from build123d import *

# Parameters (mm, degrees)
SKETCH1_R           = 3
BOSS_EXTRUDE1_DEPTH = 27
SKETCH2_R           = 4
BOSS_EXTRUDE2_DEPTH = 4
CHAMFER1_SIZE       = 2


with BuildPart() as part:
    # Sketch1 → Boss-Extrude1 (new body)
    with BuildSketch(Plane(origin=(0, 0, 0), x_dir=(0, 0, -1), z_dir=(1, 0, 0))):
        Circle(SKETCH1_R)
    extrude(amount=BOSS_EXTRUDE1_DEPTH)

    # Sketch2 → Boss-Extrude2 (add)
    with BuildSketch(Plane.ZY):
        Circle(SKETCH2_R)
    extrude(amount=BOSS_EXTRUDE2_DEPTH)

    # Chamfer1
    chamfer1_edges = [part.edges().sort_by_distance(p)[0] for p in [
        (-4, 0, -4),
    ]]
    chamfer(chamfer1_edges, length=CHAMFER1_SIZE)


solid = part.part
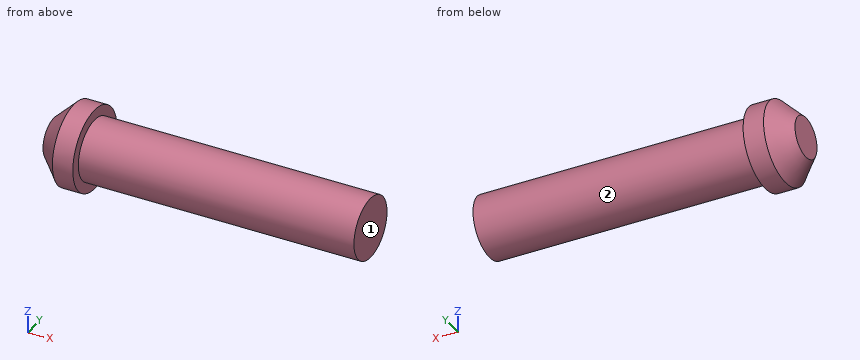
Geometry check sheet. Reference: the model listing, model coordinates, mm. Face numbers are marked on the shaded views. A direction names the side the tool comes from. Round coordinates to 2 decimals unless told otherwise and drop trailing zeros. Loops run counter-clockwise (first coordinate to the right, second up) from the corner with the lowest first, then second, coordinate; pieces in that order, holes last. Notation, with made-up numbers: (84, 22.25) - (116, 22.25) arc R7 ccw to (116, 28.25) - close; hole circle Ø8 at (-38, 32.5). An arc over 180 degrees is marked (long way). One line per question, with ' | ' between items. Start each with the question number.
1. Scan lines: line 1 (Z direction, x = -1.5, y = 3.5); line 2 (Y direction, x = -2.5, z = -1.25); line 3 (X direction, y = -2.75, z = 2.25). Record each from-to range of solid material in increasing order. Write a range as [from, to].
2. Depth check by flat-ended pin: pin 1 (1.5 mm diameter, centred on x = 19, z = 0, fed in from -Y); pin 2 (1.5 mm diameter, centred on x = 2.5, y = -3, fed in from -Z); pin 3 (4 mm diameter, centred on x = 23.5, y = 2.5, fed in from +Z). Enter the tip coordinate at first touch or a pass-through.
3. Tool access check on the marked faces 1 and 2. Record the directions out of +Z, -Z, +X, -X, +Y, -Y that give a thin tool (end or side, any length) a straight path to the whole face; none if there is none.
4. Cross-section at A-A on z = 0. Record the cut outline in (x, y), then the cut area to 3 significant figures.
5. Cross-section at C-C on x = 6. Record the cut outline in (y, z).
Taken from the geometry:
1) line 1: [-1.94, 1.94] | line 2: [-3.27, 3.27] | line 3: [-2.45, 0]
2) pin 1: y = -3 | pin 2: z = -1.98 | pin 3: z = 2.96
3) face 1: +Z, -Z, +X, +Y, -Y | face 2: +X
4) outline: (-4, -2) - (-2, -4) - (0, -4) - (0, -3) - (27, -3) - (27, 3) - (0, 3) - (0, 4) - (-2, 4) - (-4, 2) - close | area: 190 mm²
5) outline: circle Ø6 at (0, 0)
